Could you check a few things on this model? Use its own coordinates, in mm. A direction names the side the tool comes from. Coordinates: 2 decimals unless noted, no trailing zeros. Order: outer loops, then holes, each group sorted by start corner. A loop starts at its lowest first (then second) coordinate and runs counter-clockwise, first axis right, second up. Notation, with made-up numbers: (77.5, 14.5) - (114.5, 14.5) arc R18 ccw to (114.5, 38.5) - close; hole circle Ø9 at (42, 51.25). An arc over 180 degrees is marked (long way). One line per item, written item: value.
from build123d import *

# Parameters (mm, degrees)
BOSS_EXTRUDE1_DEPTH     = 50.8
SKETCH2_W               = 12.7
SKETCH2_H               = 50.8
SKETCH2_W_2             = 5.08
SKETCH2_H_2             = 41.91
BOSS_EXTRUDE2_DEPTH     = 5.08
CUT_EXTRUDE1_DEPTH      = 130.763924108
CUT_EXTRUDE1_DEPTH_BACK = 130.763924108
SKETCH5_R               = 4.0132
CUT_EXTRUDE2_DEPTH      = 12.7
BOSS_EXTRUDE3_DEPTH     = 50.8
CUT_EXTRUDE4_DEPTH      = 130.763924108
SKETCH10_W              = 5.08
SKETCH10_H              = 41.91
CUT_EXTRUDE5_DEPTH      = 127.949189836
FILLET1_R               = 2.54
FILLET2_R               = 2.54
FILLET3_R               = 2.54


with BuildPart() as part:
    # Sketch1 → Boss-Extrude1 (new body)
    with BuildSketch(Plane(origin=(0, 0, 0), x_dir=(1, 0, 0), z_dir=(0, 1, 0))):
        with BuildLine():
            Line((0, 0), (40.64, 0))
            Line((40.64, 0), (40.64, 73.66))
            Line((40.64, 73.66), (30.734, 73.66))
            ThreePointArc((30.734, 73.66), (21.082, 64.008), (11.43, 73.66))
            Line((11.43, 73.66), (0, 73.66))
            Line((0, 73.66), (0, 0))
        make_face()
        with BuildLine():
            Line((40.64, 73.66), (40.64, 0))
            Line((40.64, 0), (81.28, 0))
            Line((81.28, 0), (81.28, 73.66))
            Line((81.28, 73.66), (69.85, 73.66))
            ThreePointArc((69.85, 73.66), (60.198, 64.008), (50.546, 73.66))
            Line((50.546, 73.66), (40.64, 73.66))
        make_face()
    extrude(amount=BOSS_EXTRUDE1_DEPTH)

    # Sketch2 → Boss-Extrude2 (add)
    with BuildSketch(Plane.XY):
        with Locations((-6.35, 25.4)):
            Rectangle(SKETCH2_W, SKETCH2_H)
        with Locations((-6.35, 25.4)):
            Rectangle(SKETCH2_W_2, SKETCH2_H_2, mode=Mode.SUBTRACT)
    boss_extrude2 = extrude(amount=-BOSS_EXTRUDE2_DEPTH)

    # Mirror3: Boss-Extrude2 across plane
    add(boss_extrude2.mirror(Plane.ZY.offset(-40.64)))

    # Sketch4 → Cut-Extrude1 (cut, two sides: drawn at the far end of the back side and taken through both)
    with BuildSketch(Plane(origin=(0, 50.8, 0), x_dir=(1, 0, 0), z_dir=(0, 1, 0)).offset(-CUT_EXTRUDE1_DEPTH_BACK)):
        with BuildLine():
            Line((313.835320216, -88.467212956), (81.28, 0))
            ThreePointArc((81.28, 0), (40.64, 7.468916508), (0, 0))
            Line((0, 0), (-232.555320216, -88.467212956))
            Line((-232.555320216, -88.467212956), (-232.555320216, -586.095285833))
            Line((-232.555320216, -586.095285833), (313.835320216, -586.095285833))
            Line((313.835320216, -586.095285833), (313.835320216, -88.467212956))
        make_face()
    extrude(amount=CUT_EXTRUDE1_DEPTH + CUT_EXTRUDE1_DEPTH_BACK, mode=Mode.SUBTRACT)

    # Sketch5 → Cut-Extrude2 (cut)
    with BuildSketch(Plane(origin=(0, 0, -73.66), x_dir=(-1, 0, 0), z_dir=(0, 0, -1))):
        with Locations((-40.64, 41.91)):
            Circle(SKETCH5_R)
        with Locations(Location((-40.64, 8.89, 0), (0, 0, 180))):
            Circle(SKETCH5_R)
        with Locations((-40.64, 25.4)):
            Circle(SKETCH5_R)
    extrude(amount=-CUT_EXTRUDE2_DEPTH, mode=Mode.SUBTRACT)

    # Sketch9 → Boss-Extrude3 (add)
    with BuildSketch(Plane(origin=(0, 0, 0), x_dir=(-1, 0, 0), z_dir=(0, -1, 0))):
        Polygon((0, 5.08), (12.7, 5.08), (12.7, 10.16), (0, 16.51), (0, 8.89), align=None)
    boss_extrude3 = extrude(amount=-BOSS_EXTRUDE3_DEPTH)

    # Sketch7 → Cut-Extrude4 (cut, through all)
    with BuildSketch(Plane.XZ):
        Polygon((5.08, -16.51), (5.08, -58.42), (15.24, -58.42), align=None)
        Polygon((7.693571769, -16.51), (17.853571769, -16.51), (17.853571769, -58.42), align=None)
        Polygon((73.586428231, -16.51), (63.426428231, -16.51), (63.426428231, -58.42), align=None)
        Polygon((66.04, -58.42), (76.2, -16.51), (76.2, -58.42), align=None)
        Polygon((24.310428231, -58.42), (34.470428231, -16.51), (24.310428231, -16.51), align=None)
        Polygon((26.924, -58.42), (37.084, -16.51), (37.084, -58.42), align=None)
        Polygon((44.196, -16.51), (44.196, -58.42), (54.356, -58.42), align=None)
        Polygon((56.969571769, -58.42), (46.809571769, -16.51), (56.969571769, -16.51), align=None)
    extrude(amount=-CUT_EXTRUDE4_DEPTH, mode=Mode.SUBTRACT)

    # Sketch10 → Cut-Extrude5 (cut, through all)
    with BuildSketch(Plane.XY.offset(-5.08)):
        with Locations((-6.35, 25.4)):
            Rectangle(SKETCH10_W, SKETCH10_H)
    cut_extrude5 = extrude(amount=-CUT_EXTRUDE5_DEPTH, mode=Mode.SUBTRACT)

    # Fillet1
    fillet1_edges = [part.edges().sort_by_distance(p)[0] for p in [
        (-3.81, 46.355, -7.3025),
        (-8.89, 46.355, -6.0325),
        (-8.89, 4.445, -6.0325),
        (-3.81, 4.445, -7.3025),
    ]]
    fillet(fillet1_edges, radius=FILLET1_R - 0.0001)  # a hair under: the kernel refuses the full size

    # Mirror4: Boss-Extrude3, Cut-Extrude5 across plane
    add(boss_extrude3.mirror(Plane.ZY.offset(-40.64)))
    add(cut_extrude5.mirror(Plane.ZY.offset(-40.64)), mode=Mode.SUBTRACT)

    # Fillet2
    fillet2_edges = [part.edges().sort_by_distance(p)[0] for p in [
        (90.17, 46.355, -6.0325),
        (85.09, 46.355, -7.3025),
        (85.09, 4.445, -7.3025),
        (90.17, 4.445, -6.0325),
    ]]
    fillet(fillet2_edges, radius=FILLET2_R - 0.0001)  # a hair under: the kernel refuses the full size

    # Fillet3
    fillet3_edges = [part.edges().sort_by_distance(p)[0] for p in [
        (-3.81, 25.4, 0),
        (-8.89, 25.4, 0),
        (-4.553919486, 45.611080514, 0),
        (-8.146080514, 45.611080514, 0),
        (-8.146080514, 5.188919486, 0),
        (-4.553919486, 5.188919486, 0),
        (90.17, 25.4, 0),
        (85.09, 25.4, 0),
        (89.426080514, 45.611080514, 0),
        (85.833919486, 45.611080514, 0),
        (85.833919486, 5.188919486, 0),
        (89.426080514, 5.188919486, 0),
    ]]
    fillet(fillet3_edges, radius=FILLET3_R)


solid = part.part
Item 1: If I drill on probe 1 along Y at (x, z) = (40.64, -67.25); probe 2 along X at (y, z) = (8.89, -69.25); probe 3 along X at (y, z) = (17, -69), over which ranges is the centre line in solid material (lowest first)?
Conclusion:
probe 1: 0 to 4.88, 12.9 to 21.39, 29.41 to 37.9, 45.92 to 50.8
probe 2: 0 to 12.5, 29.67 to 36.63, 44.65 to 51.61, 68.78 to 81.28
probe 3: 0 to 12.63, 29.53 to 51.75, 68.65 to 81.28
Item 2: I want a section at C-C on x = 40.64. Please give me the cut outline in (y, z).
Conclusion:
outline: (0, -73.66) - (4.88, -73.66) - (4.88, -60.96) - (12.9, -60.96) - (12.9, -73.66) - (21.39, -73.66) - (21.39, -60.96) - (29.41, -60.96) - (29.41, -73.66) - (37.9, -73.66) - (37.9, -60.96) - (45.92, -60.96) - (45.92, -73.66) - (50.8, -73.66) - (50.8, -7.47) - (0, -7.47) - close
Item 3: I want a section at A-A on y = 31. Give the number of separate pieces and of enclosed holes in the cut face, then the cut area to 3 significant figures.
Conclusion:
separate pieces: 3
enclosed holes: 8
area: 3,780 mm²
Item 4: I want a section at B-B on x = 68. Please give me the cut outline in (y, z) (3 decimals), then the cut area to 3 significant figures.
Conclusion:
outline: (0, -67.978) - (50.8, -67.978) - (50.8, -58.42) - (0, -58.42) - close; (0, -50.335) - (50.8, -50.335) - (50.8, -39.554) - (0, -39.554) - close; (0, -16.51) - (50.8, -16.51) - (50.8, -4.146) - (0, -4.146) - close
area: 1,660 mm²
Item 5: Thinking about a two-plate mould opening in Z: for faces 5 (the face through (37.084, 25, -37)), 6 (the face through (6, 25, -73.66)), 7 (the face through (-1, 27, 0)), 8 (the face through (51.96, 25.04, -37.76)), which applies, pulls with the +Z half, pulls with the -Z half, needs draft (parallel to the pull), parting line crosses it, or undercut?
Conclusion:
face 5: undercut
face 6: pulls with the -Z half
face 7: pulls with the +Z half
face 8: undercut
Item 6: For faces 1 (the face through (84.4, 25.1, -0.8)), 2 (the face through (-4.534, 5.209, -8.657)), 3 (the face through (41, 25, -60.96)), 4 (the face through (49.347, 25.044, -37.758)), which set-ups out of +Z, -Z, +X, -X, +Y, -Y let a thin tool reach every point of the face, with its end or its side?
Conclusion:
face 1: +Z
face 2: +Z, -Z
face 3: -Z
face 4: +Y, -Y
Item 7: I'm going to push flat-ended pins straight in: pin 1 Ø6 at (y, z) = (16, -32.5) entering from -X; pin 2 Ø2 at (y, z) = (19, -65.5) entering from +X; pin 3 Ø3 at (x, y) = (69, 13.5) entering from +Z. Where does each tip first touch, or does it pass through?
Conclusion:
pin 1: x = 0
pin 2: x = 81.28
pin 3: z = -3.5
